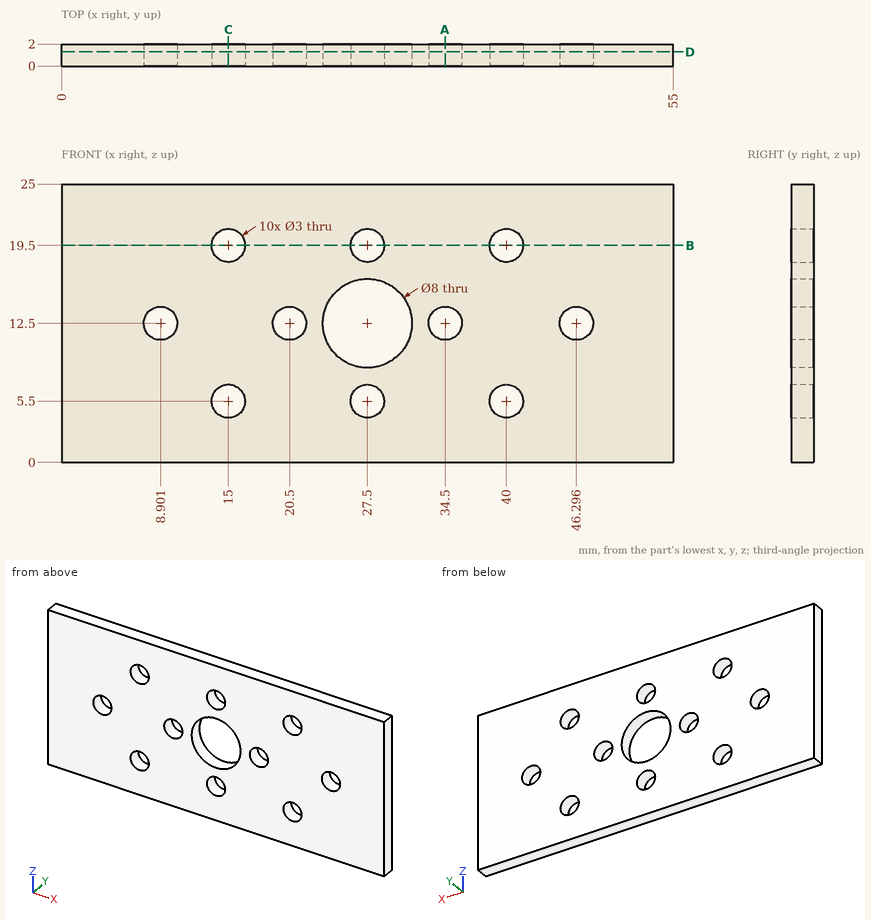
The figure shows three views and two pictorial views of one solid part (mm, origin at its lowest corner). Answer the questions. Round coordinates to 2 decimals unless told otherwise and drop trailing zeros. Write each loop counter-clockwise with the first axis right and the second up, starting at its lowest first coordinate (ties: lowest second). Pieces come first, ordered by that corner, then holes. Notation, with made-up numbers: (-20, 79.5) -> (15, 79.5) arc R11 ccw to (15, 91.5) -> close; hole circle Ø5 at (27.5, 22.5). An arc over 180 degrees is marked (long way). Answer as a JSON object with one key per item and string values. Group by question number.
Q1. Section B-B (z = 19.5) is taken. Write down the section's boundary in (x, y).
Q2. Straight lines are drawn through the part: line 1 along X through (y, z) = (0.6, 12.5); line 2 along X through (y, z) = (1.2, 5.5); line 3 along Z through (x, y) = (28, 0.4) (1 decimal). For each, find the intervals that lie inside material, in ascending order.
Q3. Section C-C (x = 15) is taken. Write down the section's boundary in (y, z), plus the area to 3 significant figures.
Q4. Section A-A (x = 34.5) is taken. Write down the section's boundary in (y, z), plus the area to 3 significant figures.
Q5. Section D-D (y = 1.3) is taken. Count the separate pieces of the cut face and the enclosed holes in it, plus the area to 3 significant figures.
Check values:
{
 "1": {"outline": "(0, 0) -> (13.5, 0) -> (13.5, 2) -> (0, 2) -> close; (16.5, 0) -> (26, 0) -> (26, 2) -> (16.5, 2) -> close; (29, 0) -> (38.5, 0) -> (38.5, 2) -> (29, 2) -> close; (41.5, 0) -> (55, 0) -> (55, 2) -> (41.5, 2) -> close"},
 "2": {"line 1": "0 to 7.4, 10.4 to 19, 22 to 23.5, 31.5 to 33, 36 to 44.8, 47.8 to 55", "line 2": "0 to 13.5, 16.5 to 26, 29 to 38.5, 41.5 to 55", "line 3": "0 to 4.1, 6.9 to 8.5, 16.5 to 18.1, 20.9 to 25"},
 "3": {"outline": "(0, 0) -> (2, 0) -> (2, 4) -> (0, 4) -> close; (0, 7) -> (2, 7) -> (2, 18) -> (0, 18) -> close; (0, 21) -> (2, 21) -> (2, 25) -> (0, 25) -> close", "area": "38.0 mm^2"},
 "4": {"outline": "(0, 0) -> (2, 0) -> (2, 11) -> (0, 11) -> close; (0, 14) -> (2, 14) -> (2, 25) -> (0, 25) -> close", "area": "44.0 mm^2"},
 "5": {"separate pieces": "1", "enclosed holes": "11", "area": "1,250 mm^2"}
}
